Solid Edge part; units mm, degrees
sketch "Sketch1" plane through (0, 0, 0) normal (0, 0, 1) x (1, 0, 0)
  line L0 (-250, -300) -> (250, -300)
  line L1 (250, -300) -> (250, 300)
  line L2 (250, 300) -> (-250, 300)
  line L3 (-250, 300) -> (-250, -300)
  dimension "D1" = 250
  dimension "D2" = 250
extrude "Protrusion1" add sketch "Sketch1" along normal blind 1100
sketch "Sketch2" plane through (0, 0, 1100) normal (0, 0, 1) x (1, 0, 0)
  circle A0 centre (0, 0) radius 100
extrude "Cutout1" cut sketch "Sketch2" against normal up to next
sketch "Sketch3" plane through (250, 0, 550) normal (1, 0, 0) x (0, 1, 0)
  line L0 (-192.0896, 299.5224) -> (207.9104, 299.5224)
  line L1 (207.9104, 299.5224) -> (207.9104, -100.4776)
  line L2 (207.9104, -100.4776) -> (-192.0896, -100.4776)
  line L3 (-192.0896, -100.4776) -> (-192.0896, 299.5224)
  dimension "D1" = 192.0896
  dimension "D2" = 207.9104
extrude "Protrusion2" add sketch "Sketch3" along normal blind 900
Source: CAD feature listing. Evaluate the final solid. Frame: model axes, mm. A direction names the side the tool comes from. Give positions to 0.01 mm unless a question says otherwise; leave off trailing zeros. Write each loop counter-clockwise with the first axis right and the second up, starting at its lowest first coordinate (ties: lowest second). Pieces come first, ordered by that corner, then holes.
1. Pull-direction query (X, two-part tool) for faces 1 (the face through (3, 300, 542)), 2 (the face through (-250, 4, 542)), 3 (the face through (95.38, 30.04, 557.7)); classes: +X half, -X half, draft (parallel to the pull), parting line (faces both ways), or undercut.
2. First-contact query: pin 1 (1 mm diameter, centred on y = -16.5, z = 368.5, fed in from +X); pin 2 (12 mm diameter, centred on x = 948.5, y = 171, fed in from -Z); pin 3 (5 mm diameter, centred on x = 690, y = 87.5, fed in from +Z). Flat tips, straight axial feed; report the tip coordinate or a pass-through.
3. Section query D-D (y = -214). Return the cut outline in (x, z), then the cut area to 3 significant figures.
4. Material intervals for line 1 along Y through (x, z) = (0, 280); line 2 along Z through (x, y) = (565, -157); line 3 along Y through (x, z) = (298, 810), sorted ascending.
5. Section query B-B (y = 0). Return the cut outline in (x, z), then the cut area to 3 significant figures.
6. Access query for faces 4 (the face through (-3, -300, 542)), 5 (the face through (694, -192.09, 647)), 6 (the face through (694, 11, 449.522)), 7 (the face through (694, 207.91, 652)), 8 (the face through (694, 5, 849.522)). Directions: +Z, -Z, +X, -X, +Y, -Y. A direction counts if a zero-diameter tool reaches every point of the face in a straight line with its end or side. Return the directions, or none.
7. Section query C-C (z = 602.5). Return the cut outline in (x, y).
8. Section query A-A (x = 0). Return the cut outline in (y, z).
Output values:
1. face 1: draft
1. face 2: -X half
1. face 3: undercut
2. pin 1: stops at x = 250
2. pin 2: stops at z = 449.52
2. pin 3: stops at z = 849.52
3. outline: (-250, 0) - (250, 0) - (250, 1100) - (-250, 1100) - close
3. area: 550,000 mm2
4. line 1: y = -300 to -100, 100 to 300
4. line 2: z = 449.52 to 849.52
4. line 3: y = -192.09 to 207.91
5. outline: (-250, 0) - (-100, 0) - (-100, 1100) - (-250, 1100) - close; (100, 0) - (250, 0) - (250, 449.52) - (1150, 449.52) - (1150, 849.52) - (250, 849.52) - (250, 1100) - (100, 1100) - close
5. area: 690,000 mm2
6. face 4: +Z, -Z, +X, -X, -Y
6. face 5: +Z, -Z, +X, -Y
6. face 6: -Z, +X, +Y, -Y
6. face 7: +Z, -Z, +X, +Y
6. face 8: +Z, +X, +Y, -Y
7. outline: (-250, -300) - (250, -300) - (250, -192.09) - (1150, -192.09) - (1150, 207.91) - (250, 207.91) - (250, 300) - (-250, 300) - close; hole circle Ø200 at (0, 0)
8. outline: (-300, 0) - (-100, 0) - (-100, 1100) - (-300, 1100) - close; (100, 0) - (300, 0) - (300, 1100) - (100, 1100) - close
